```python
from build123d import *

# Parameters (mm, degrees)
F1_DEPTH = 25


with BuildPart() as f1:
    # F0 (on Front) → F1 (new body)
    with BuildSketch(Plane.XZ):
        with BuildLine():
            ThreePointArc((31.524628, -41.74067), (34.482234, -39.971165), (37.336944, -38.040047))
            ThreePointArc((37.336944, -38.040047), (40.188741, -35.865425), (42.910032, -33.52955))
            Line((42.910032, -33.52955), (42.910032, 39.535794))
            ThreePointArc((42.910032, 39.535794), (22.83568, 50.899702), (0, 54.163095))
            ThreePointArc((0, 54.163095), (-22.83568, 50.899702), (-42.910032, 39.535794))
            Line((-42.910032, 39.535794), (-42.910032, -33.52955))
            ThreePointArc((-42.910032, -33.52955), (-40.188741, -35.865425), (-37.336944, -38.040047))
            ThreePointArc((-37.336944, -38.040047), (-35.258682, -39.468633), (-33.124044, -40.81152))
            ThreePointArc((-33.124044, -40.81152), (-17.185862, -47.571204), (0, -49.660496))
            ThreePointArc((0, -49.660496), (16.290558, -47.803241), (31.524628, -41.74067))
        make_face()
        with BuildLine():
            ThreePointArc((31.285256, -16.673503), (-0.778877, -27.258788), (-31.63917, -13.554801))
            ThreePointArc((-31.63917, -13.554801), (-0.177021, -15.115437), (31.285256, -16.673503))
        make_face(mode=Mode.SUBTRACT)
        with BuildLine():
            Line((-25.309497, 11.731247), (-28.83604, 11.731247))
            Line((-28.83604, 11.731247), (-28.83604, 24.857815))
            ThreePointArc((-28.83604, 24.857815), (-22.860512, 28.786769), (-16.884984, 24.857815))
            Line((-16.884984, 24.857815), (-16.884984, 11.731247))
            Line((-16.884984, 11.731247), (-20.711496, 11.731247))
            Line((-20.711496, 11.731247), (-25.309497, 11.731247))
        make_face(mode=Mode.SUBTRACT)
        with BuildLine():
            Line((20.711496, 11.731247), (16.884984, 11.731247))
            Line((16.884984, 11.731247), (16.884984, 24.857815))
            ThreePointArc((16.884984, 24.857815), (22.860512, 28.786769), (28.83604, 24.857815))
            Line((28.83604, 24.857815), (28.83604, 11.731247))
            Line((28.83604, 11.731247), (25.309497, 11.731247))
            Line((25.309497, 11.731247), (20.711496, 11.731247))
        make_face(mode=Mode.SUBTRACT)
        with BuildLine():
            Line((-25.309497, 18.588411), (-25.309497, 11.731247))
            Line((-25.309497, 11.731247), (-20.711496, 11.731247))
            Line((-20.711496, 11.731247), (-20.711496, 18.588411))
            ThreePointArc((-20.711496, 18.588411), (-23.010497, 20.887411), (-25.309497, 18.588411))
        make_face()
        with BuildLine():
            Line((20.711496, 18.588411), (20.711496, 11.731247))
            Line((20.711496, 11.731247), (25.309497, 11.731247))
            Line((25.309497, 11.731247), (25.309497, 18.588411))
            ThreePointArc((25.309497, 18.588411), (23.010497, 20.887411), (20.711496, 18.588411))
        make_face()
        with BuildLine():
            Line((-33.124044, -62.074588), (-33.124044, -40.81152))
            ThreePointArc((-33.124044, -40.81152), (-35.258682, -39.468633), (-37.336944, -38.040047))
            Line((-37.336944, -38.040047), (-37.336944, -62.185542))
            Line((-37.336944, -62.185542), (-33.124044, -62.074588))
        make_face()
        with BuildLine():
            Line((31.524628, -64.615463), (37.336944, -62.185542))
            Line((37.336944, -62.185542), (37.336944, -38.040047))
            ThreePointArc((37.336944, -38.040047), (34.482234, -39.971165), (31.524628, -41.74067))
            Line((31.524628, -41.74067), (31.524628, -64.615463))
        make_face()
    extrude(amount=F1_DEPTH)


solid = f1.part
```
CAD build for the part. Positions are in the model's coordinates, mm. A direction names the side the tool comes from. Round coordinates to 2 decimals unless told otherwise and drop trailing zeros. Order: outer loops, then holes, each group sorted by start corner. A loop starts at its lowest first (then second) coordinate and runs counter-clockwise, first axis right, second up. Notation, with made-up numbers: (37.25, 86.5) - (46.25, 86.5) arc R27 ccw to (46.25, 111.5) - close; hole circle Ø1 at (28.5, -37.5). An arc over 180 degrees is marked (long way). Answer as CSV lines item,"result". Start each with the question number.
1. Pin check, flat tips, straight feed: pin 1 (3 mm diameter, centred on x = 22.5, y = -12.5, fed in from +Z); pin 2 (1.8 mm diameter, centred on x = -28, y = -9, fed in from +Z); pin 3 (1.5 mm diameter, centred on y = -6.5, z = -49.5, fed in from +X); pin 4 (12 mm diameter, centred on x = 25, z = -28.5, fed in from +Y). Stop position of each tip, or through.
2. Saw through at B-B, the plane z = -22. Write the cut outline in (x, y).
3. Tool access for faces 4 (the face through (31.525, -12, -53)), 5 (the face through (-0.617, -12.325, -15.094)), 6 (the face through (34.39, -12.325, -63.418)): list every direction of +Z, -Z, +X, -X, +Y, -Y with a clear straight run to the whole face (end or side of a thin tool).
4. Saw through at C-C, the plane y = -17.75. Count the separate pieces of the cut face and the enclosed holes in it, and give its area (3 significant figures).
5. Pull direction Z, two halves, no side cores. Call faces 1 (the face through (-33.124, -12, -52)), 2 (the face through (-40.23, -12.32, -35.83)), 3 (the face through (-22.96, -12.325, 20.887)): +Z half, -Z half, draft (parallel to the pull), parting line (faces both ways), or undercut.
6. Drill centre lines: L1, parallel to Z at x = -17.5, y = -12.25; L2, parallel to X at y = -23.5, z = 17; L3, parallel to Z at x = 11, y = -19.25. Where is each one in solid material? Low to high. Write a range as [from, to].
7. Saw through at D-D, the plane z = -47.5. Write the cut outline in (x, y).
8. Saw through at A-A, the plane x = -8. Write the cut outline in (y, z), and give its area (3 significant figures).
Model answer:
1,pin 1,"stops at z = 51.49"
1,pin 2,"stops at z = 49.27"
1,pin 3,"stops at x = 37.34"
1,pin 4,"stops at y = 0"
2,outline,"(-42.91, -25) - (-20.14, -25) - (-20.14, 0) - (-42.91, 0) - close; (23.23, -25) - (42.91, -25) - (42.91, 0) - (23.23, 0) - close"
3,face 4,"-Z, +Y, -Y"
3,face 5,"+Y, -Y"
3,face 6,"-Z, +X, +Y, -Y"
4,separate pieces,"1"
4,enclosed holes,"3"
4,area,"7,530 mm²"
5,face 1,"draft"
5,face 2,"-Z half"
5,face 3,"undercut"
6,L1,"z = [-47.49, -23.28], [-14.26, 11.73], [25.97, 52.46]"
6,L2,"x = [-42.91, -28.84], [-25.31, -20.71], [-16.88, 16.88], [20.71, 25.31], [28.84, 42.91]"
6,L3,"z = [-48.89, -26.35], [-15.67, 53.68]"
7,outline,"(-37.34, -25) - (-33.12, -25) - (-33.12, 0) - (-37.34, 0) - close; (-17.45, -25) - (17.45, -25) - (17.45, 0) - (-17.45, 0) - close; (31.52, -25) - (37.34, -25) - (37.34, 0) - (31.52, 0) - close"
8,outline,"(-25, -49.3) - (0, -49.3) - (0, -26.33) - (-25, -26.33) - close; (-25, -14.73) - (0, -14.73) - (0, 54.01) - (-25, 54.01) - close"
8,area,"2,290 mm²"
